from build123d import *

# Parameters (mm, degrees)
BASE_EXTRUDE_DEPTH             = 12.7
F_9_16_0_5625_DIAMETER_HOLE1_D = 14.2875
CUT_EXTRUDE1_DEPTH             = 13.7
BOSS_EXTRUDE1_DEPTH            = 25.4
F_1_2_20_TAPPED_HOLE1_D        = 12.7
CUT_EXTRUDE2_DEPTH             = 39.1
CUT_EXTRUDE3_DEPTH             = 39.1
F_1_2_20_TAPPED_HOLE2_D        = 12.7
CUT_EXTRUDE4_DEPTH             = 25.4


with BuildPart() as part:
    # Sketch1 → Base-Extrude (new body)
    with BuildSketch(Plane.XY):
        Polygon((58.12164787, 111.098459585), (-37.201684746, 66.648459585), (-37.201684746, -66.701540415), (264.657388756, -66.701540415), (264.657388756, 66.648459585), (169.334056139, 111.098459585), align=None)
    extrude(amount=BASE_EXTRUDE_DEPTH)

    # 9/16 (0.5625) Diameter Hole1 (through all)
    with Locations(Plane.XY.offset(12.7)):
        with Locations((251.957388756, -9.551540415), (251.957388756, 41.248459585)):
            f_9_16_0_5625_diameter_hole1 = Hole(F_9_16_0_5625_DIAMETER_HOLE1_D / 2)

    # Sketch8 → Cut-Extrude1 (cut, through all)
    with BuildSketch(Plane.XY.offset(12.7)):
        with BuildLine():
            Line((-12.371439248, -66.701540415), (239.908029755, -66.701540415))
            Line((239.908029755, -66.701540415), (130.710820593, -10.795488361))
            ThreePointArc((130.710820593, -10.795488361), (119.603489866, -8.008935492), (108.401043329, -10.384406895))
            Line((108.401043329, -10.384406895), (-12.371439248, -66.701540415))
        make_face()
    extrude(amount=-CUT_EXTRUDE1_DEPTH, mode=Mode.SUBTRACT)

    # Mirror3: 9/16 (0.5625) Diameter Hole1 across plane
    add(f_9_16_0_5625_diameter_hole1.mirror(Plane(origin=(113.768295254, 0, 0), x_dir=(0, 0, 1), z_dir=(1, 0, 0))), mode=Mode.SUBTRACT)

    # Sketch10 → Boss-Extrude1 (add)
    with BuildSketch(Plane(origin=(0, 0, 0), x_dir=(-1, 0, 0), z_dir=(0, 0, -1))):
        Polygon((-169.334056139, 111.098459585), (-58.12164787, 111.098459585), (33.824515248, 68.223259585), (-261.280219258, 68.223259585), align=None)
    extrude(amount=BOSS_EXTRUDE1_DEPTH)

    # 1/2-20 Tapped Hole1 (through all)
    with Locations(Plane(origin=(0, 111.098459585, 0), x_dir=(-1, 0, 0), z_dir=(0, 1, 0))):
        with Locations((-113.69684787, -12.7)):
            Hole(F_1_2_20_TAPPED_HOLE1_D / 2)

    # Sketch13 → Cut-Extrude2 (cut, through all)
    with BuildSketch(Plane.XY.offset(12.7)):
        with BuildLine():
            Line((250.369888756, -2.407790415), (253.544888756, -2.407790415))
            ThreePointArc((253.544888756, -2.407790415), (260.688638756, -9.551540415), (253.544888756, -16.695290415))
            Line((253.544888756, -16.695290415), (250.369888756, -16.695290415))
            ThreePointArc((250.369888756, -16.695290415), (243.226138756, -9.551540415), (250.369888756, -2.407790415))
        make_face()
    cut_extrude2 = extrude(amount=-CUT_EXTRUDE2_DEPTH, mode=Mode.SUBTRACT)

    # Sketch14 → Cut-Extrude3 (cut, through all)
    with BuildSketch(Plane.XY.offset(12.7)):
        with BuildLine():
            Line((253.544888756, 48.392209585), (250.369888756, 48.392209585))
            ThreePointArc((250.369888756, 48.392209585), (243.226138756, 41.248459585), (250.369888756, 34.104709585))
            Line((250.369888756, 34.104709585), (253.544888756, 34.104709585))
            ThreePointArc((253.544888756, 34.104709585), (260.688638756, 41.248459585), (253.544888756, 48.392209585))
        make_face()
    cut_extrude3 = extrude(amount=-CUT_EXTRUDE3_DEPTH, mode=Mode.SUBTRACT)

    # Mirror4: Cut-Extrude2, Cut-Extrude3 across plane
    add(cut_extrude2.mirror(Plane(origin=(113.768295254, 0, 0), x_dir=(0, 0, 1), z_dir=(1, 0, 0))), mode=Mode.SUBTRACT)
    add(cut_extrude3.mirror(Plane(origin=(113.768295254, 0, 0), x_dir=(0, 0, 1), z_dir=(1, 0, 0))), mode=Mode.SUBTRACT)

    # 1/2-20 Tapped Hole2 (through all)
    with Locations(Plane.XY.offset(12.7)):
        with Locations((38.998315254, 41.248459585), (188.457388756, 41.248459585)):
            Hole(F_1_2_20_TAPPED_HOLE2_D / 2)

    # Sketch17 → Cut-Extrude4 (cut)
    with BuildSketch(Plane(origin=(0, 0, -25.4), x_dir=(-1, 0, 0), z_dir=(0, 0, -1))):
        with BuildLine():
            Line((-129.602852005, 68.223259585), (-97.852852005, 68.223259585))
            Line((-97.852852005, 68.223259585), (-97.852852005, 88.848059585))
            ThreePointArc((-97.852852005, 88.848059585), (-99.251475703, 92.224635886), (-102.628052005, 93.623259585))
            Line((-102.628052005, 93.623259585), (-124.827652005, 93.623259585))
            ThreePointArc((-124.827652005, 93.623259585), (-128.204228306, 92.224635886), (-129.602852005, 88.848059585))
            Line((-129.602852005, 88.848059585), (-129.602852005, 68.223259585))
        make_face()
    extrude(amount=-CUT_EXTRUDE4_DEPTH, mode=Mode.SUBTRACT)


solid = part.part
Design review of the part built by this model. Coordinates are the model's own, in mm. A direction names the side the tool comes from. Coordinates: 2 decimals unless noted, no trailing zeros. Loops run counter-clockwise (first coordinate to the right, second up) from the corner with the lowest first, then second, coordinate; pieces in that order, holes last. Notation, with made-up numbers: (50.5, 79.25) -> (91.5, 79.25) arc R15 cw to (91.5, 94.25) -> close; hole circle Ø2 at (-15, 27). An arc over 180 degrees is marked (long way). Use a Markdown table: item, result. Add a question column.
Item 1: Machinability: for faces 1 (the flat face through (112, 95, -25.4)), 2 (the cylindrical face through (-15.69, -9.71, 6.44)), 3 (the flat face through (97.853, 78, -13)), which of the approach directions +Z, -Z, +X, -X, +Y, -Y give a long, thin tool a straight path to every point of the face, cutting with its end or side? Answer none if there is none.
Item 2: We need section B-B, the plane y = -34.5. Write out the cut boundary in (x, z), and give its area (3 significant figures).
Item 3: We need section A-A, the plane z = -12.7. Write out the cut boundary in (x, y).
Item 4: We need section C-C, the plane z = 6.5. Write out the cut boundary in (x, y), and give its area (3 significant figures).
Item 5: Wall thickness on L1, parallel to Y at x = 70.5, z = -20; L2, parallel to X at y = 100, z = -12; L3, parallel to Z at x = 219, y = -27.5: over which ranges is each line inside the solid? List them lowest first. Write a range as from..to.
Item 6: Clearance check with flat-ended pins moving along their axes: P1, Ø2.5, axis at x = 251.5, z = 5, coming from the +Y side; P2, Ø3.5, axis at x = -25, z = 4.5, coming from the +Y side; P3, Ø3.5, axis at x = 251.5, z = 9, coming from the +Y side. State where each tip first meets the part, or that it passes through.
Item 7: We need section D-D, the plane x = 138.5. Write out the cut boundary in (y, z), and give its area (3 significant figures).
Item 8: The part is to be moulded in two halves that separate along X. For faces 4 (the flat face through (111, 93.623, -19)), 5 (the flat face through (264.657, -1, 6)), 6 (the flat face through (115, 111.098, -6)), say which applies: +X half, -X half, draft (parallel to the pull), parting line (faces both ways), or undercut.
Numbers:
| question | item | result |
|---|---|---|
| 1 | face 1 | -Z, +X, -X, +Y, -Y |
| 1 | face 2 | +Z, -Z |
| 1 | face 3 | -Z, -Y |
| 2 | outline | (-37.2, 0) -> (56.68, 0) -> (56.68, 12.7) -> (-37.2, 12.7) -> close; (177.01, 0) -> (264.66, 0) -> (264.66, 12.7) -> (177.01, 12.7) -> close |
| 2 | area | 2,310 mm^2 |
| 3 | outline | (-33.82, 68.22) -> (97.85, 68.22) -> (97.85, 88.85) arc R4.78 cw to (102.63, 93.62) -> (107.35, 93.62) -> (107.35, 111.1) -> (58.12, 111.1) -> close; (120.05, 93.62) -> (124.83, 93.62) arc R4.78 cw to (129.6, 88.85) -> (129.6, 68.22) -> (261.28, 68.22) -> (169.33, 111.1) -> (120.05, 111.1) -> close |
| 4 | outline | (-37.2, -66.7) -> (-12.37, -66.7) -> (108.4, -10.38) arc R25.4 cw to (130.71, -10.8) -> (239.91, -66.7) -> (264.66, -66.7) -> (264.66, 66.65) -> (169.33, 111.1) -> (58.12, 111.1) -> (-37.2, 66.65) -> close; hole (-26.01, -16.7) -> (-22.83, -16.7) arc R7.14 ccw to (-22.83, -2.41) -> (-26.01, -2.41) arc R7.14 ccw to start; hole (-26.01, 34.1) -> (-22.83, 34.1) arc R7.14 ccw to (-22.83, 48.39) -> (-26.01, 48.39) arc R7.14 ccw to start; hole circle Ø12.7 at (39, 41.25); hole circle Ø12.7 at (188.46, 41.25); hole (250.37, -16.7) -> (253.54, -16.7) arc R7.14 ccw to (253.54, -2.41) -> (250.37, -2.41) arc R7.14 ccw to start; hole (250.37, 34.1) -> (253.54, 34.1) arc R7.14 ccw to (253.54, 48.39) -> (250.37, 48.39) arc R7.14 ccw to start |
| 4 | area | 40,600 mm^2 |
| 5 | L1 | y = 68.22..111.1 |
| 5 | L2 | x = 34.32..107.39, 120.01..193.13 |
| 5 | L3 | z = 0..12.7 |
| 6 | P1 | stops at y = 73.37 |
| 6 | P2 | stops at y = 73.15 |
| 6 | P3 | stops at y = 73.6 |
| 7 | outline | (-14.78, 0) -> (68.22, 0) -> (68.22, -25.4) -> (111.1, -25.4) -> (111.1, 12.7) -> (-14.78, 12.7) -> close |
| 7 | area | 2,690 mm^2 |
| 8 | face 4 | undercut |
| 8 | face 5 | +X half |
| 8 | face 6 | draft |
